Build history of the part. All positions in model axes, mm. Face numbers are marked on the shaded views. Give positions to 0.01 mm unless a question says otherwise; leave off trailing zeros. Write each loop counter-clockwise with the first axis right and the second up, starting at its lowest first coordinate (ties: lowest second). Pieces come first, ordered by that corner, then holes. Notation, with made-up numbers: (-31, -36) -> (1, -36) arc R22 cw to (1, -9) -> close; hole circle Ø10 at (24, -22.75). An arc over 180 degrees is marked (long way). Put each result on its own line as item: value. Start each with the question number.
Item 1: Drill centre lines: line 1 along Z through (x, y) = (31.5, -17.5); line 2 along Z through (x, y) = (2, -64); line 3 along X through (y, z) = (-63.5, 12.5). Where is each one in solid material? Low to high.
Item 2: Flat gauge pin, fed straight in: pin 1 Ø5 at (x, y) = (3.5, -28) entering from +Z. Where does the tip first touch, or does it go through?
Item 3: Slice it at B-B, the plane y = -49.5. List the corners of the cut face in (x, z), plus the area to 3 significant figures.
Item 4: Slice it at C-C, the plane x = 3. List the corners of the cut face in (y, z).
Item 5: Two-plate mould, pull along Z, no slides. Class the marked faces 1, 2, 3 and 4: pulls with the +Z half, pulls with the -Z half, needs draft (parallel to the pull), parting line crosses it, or undercut.
Item 6: Slice it at A-A, the plane x = 32. List the corners of the cut face in (y, z).
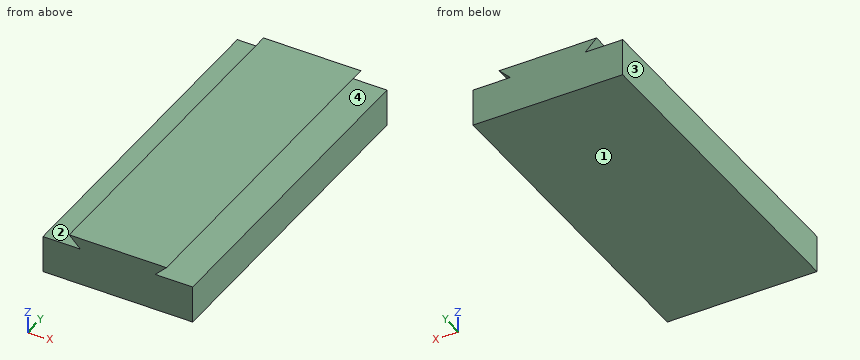
```python
from build123d import *

# Parameters (mm, degrees)
SKETCH_1_W      = 40
SKETCH_1_H      = 90
EXTRUDE_1_DEPTH = 10
EXTRUDE_2_DEPTH = 90


with BuildPart() as part:
    # 草图1 → 凸台-拉伸1 (new body)
    with BuildSketch(Plane.XY):
        with Locations((20, -45)):
            Rectangle(SKETCH_1_W, SKETCH_1_H)
    extrude(amount=EXTRUDE_1_DEPTH)

    # 草图2 → 凸台-拉伸2 (add)
    with BuildSketch(Plane.XZ.offset(90)):
        Polygon((10, 10), (7, 13), (33, 13), (30, 10), align=None)
    extrude(amount=-EXTRUDE_2_DEPTH)


solid = part.part
```
Values follow:
1. line 1: 0 to 10, 11.5 to 13
1. line 2: 0 to 10
1. line 3: 7.5 to 32.5
2. pin 1: z = 10
3. outline: (0, 0) -> (40, 0) -> (40, 10) -> (30, 10) -> (33, 13) -> (7, 13) -> (10, 10) -> (0, 10) -> close
3. area: 469 mm2
4. outline: (-90, 0) -> (0, 0) -> (0, 10) -> (-90, 10) -> close
5. face 1: pulls with the -Z half
5. face 2: undercut
5. face 3: needs draft
5. face 4: undercut
6. outline: (-90, 0) -> (0, 0) -> (0, 10) -> (-90, 10) -> close; (-90, 12) -> (0, 12) -> (0, 13) -> (-90, 13) -> close
